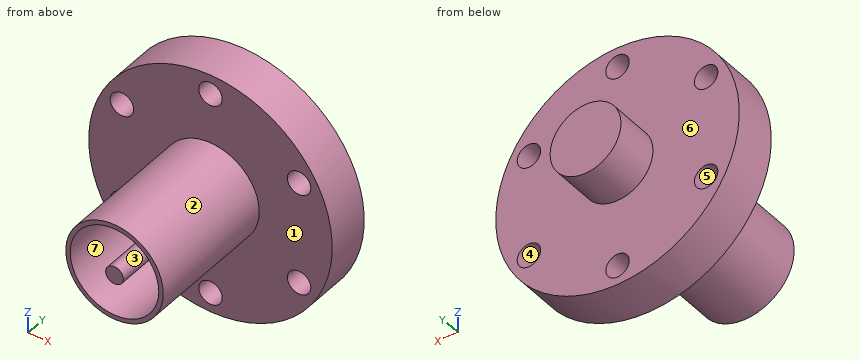
```python
from build123d import *

# Parameters (mm, degrees)
SKETCH1_R           = 34.925
EXTRUDE1_DEPTH      = 12.7
SKETCH3_R           = 3.3655
CUT_EXTRUDE2_DEPTH  = 12.7
CIRPATTERN1_COUNT   = 6
SKETCH6_R           = 10.16
EXTRUDE2_DEPTH      = 12.7
SKETCH7_R           = 13.97
SKETCH7_R_2         = 12.7
EXTRUDE_THIN2_DEPTH = 38.1
SKETCH8_R           = 2.54
EXTRUDE4_DEPTH      = 38.1


with BuildPart() as part:
    # Sketch1 → Extrude1 (new body)
    with BuildSketch(Plane(origin=(0, 0, 0), x_dir=(1, 0, 0), z_dir=(0, 1, 0))):
        with Locations(Location((0, 0, 0), (0, 0, 270))):
            Circle(SKETCH1_R)
    extrude(amount=EXTRUDE1_DEPTH)

    # Sketch3 → Cut-Extrude2 (cut)
    with BuildSketch(Plane(origin=(0, 0, 0), x_dir=(1, 0, 0), z_dir=(0, 1, 0))):
        with Locations(Location((0, 29.337, 0), (0, 0, 270))):
            Circle(SKETCH3_R)
    cut_extrude2 = extrude(amount=CUT_EXTRUDE2_DEPTH, mode=Mode.SUBTRACT)

    # CirPattern1: Cut-Extrude2 ×6 about axis
    cirpattern1_axis = Axis((0, 0, 0), (0, 1, 0))
    for i in range(1, CIRPATTERN1_COUNT):
        add(cut_extrude2.rotate(cirpattern1_axis, i * 360 / CIRPATTERN1_COUNT), mode=Mode.SUBTRACT)

    # Sketch6 → Extrude2 (add)
    with BuildSketch(Plane(origin=(0, 12.7, 0), x_dir=(-1, 0, 0), z_dir=(0, 1, 0))):
        with Locations(Location((0, 0, 0), (0, 0, 90))):
            Circle(SKETCH6_R)
    extrude(amount=EXTRUDE2_DEPTH)

    # Sketch7 → Extrude-Thin2 (add)
    with BuildSketch(Plane.XZ):
        with Locations((0, 0.982903874)):
            Circle(SKETCH7_R)
        with Locations((0, 0.982903874)):
            Circle(SKETCH7_R_2, mode=Mode.SUBTRACT)
    extrude(amount=EXTRUDE_THIN2_DEPTH)

    # Sketch8 → Extrude4 (add)
    with BuildSketch(Plane.XZ):
        with Locations(Location((0, 0, 0), (0, 0, 90))):
            Circle(SKETCH8_R)
    extrude(amount=EXTRUDE4_DEPTH)


solid = part.part
```
CAD build for the part. Positions are in the model's coordinates, mm. Face numbers are marked on the shaded views. A direction names the side the tool comes from. Give positions to 0.01 mm unless a question says otherwise; leave off trailing zeros. Order: outer loops, then holes, each group sorted by start corner. A loop starts at its lowest first (then second) coordinate and runs counter-clockwise, first axis right, second up.
(1) Mould opens along X. For the marked faces 1, 2, 3 and 4 say: released by +X, released by -X, zero draft, split by the parting line, or undercut.
(2) Tool access for the marked faces 5, 6 and 7: list every direction of +Z, -Z, +X, -X, +Y, -Y with a clear straight run to the whole face (end or side of a thin tool).
(3) Drill centre lines: L1, parallel to Z at x = 0.5, y = 12; L2, parallel to X at y = -25, z = -9; L3, parallel to Y at x = -6.5, z = -25. Where is each one in solid material? Low to high.
(4) Saw through at C-C, the plane z = -15. Give the cut face in (x, y), then the cut area to 3 significant figures.
(5) Saw through at B-B, the plane y = 11.5. State how many separate pieces and enclosed holes the cut face has, then the cut area to 3 significant figures.
(6) Saw through at D-D, the plane y = -17.5. Give the cut face in (x, z), then the cut area to 3 significant figures.
(7) Saw through at A-A, the plane x = 0. Give the cut face in (y, z) (1 decimal).
(8) Flat gauge pins, fed straight in: pin 1 (7.5 mm diameter, centred on x = 25.41, z = -14.67, fed in from +Y); pin 2 (6 mm diameter, centred on x = 19.5, y = 5.5, fed in from +Z); pin 3 (2 mm diameter, centred on x = -22.5, y = -0.5, fed in from -Z); pin 4 (4 mm diameter, centred on x = -25.41, z = -14.67, fed in from -Y). Where does each tip first touch, or does it go through?
Results found:
1. face 1: zero draft
1. face 2: split by the parting line
1. face 3: undercut
1. face 4: undercut
2. face 5: +Y, -Y
2. face 6: +Y
2. face 7: -Y
3. L1: z = -34.92 to -32.67, -26.01 to 26.01, 32.67 to 34.92
3. L2: x = -9.77 to -7.85, 7.85 to 9.77
3. L3: y = 0 to 12.7
4. outline: (-31.54, 0) - (-28.76, 0) - (-28.76, 12.7) - (-31.54, 12.7) - close; (-22.06, 0) - (22.06, 0) - (22.06, 12.7) - (-22.06, 12.7) - close; (28.76, 0) - (31.54, 0) - (31.54, 12.7) - (28.76, 12.7) - close
4. area: 631 mm2
5. separate pieces: 1
5. enclosed holes: 6
5. area: 3,620 mm2
6. outline: circle Ø27.94 at (0, 0.98); circle Ø5.08 at (0, 0); hole circle Ø25.4 at (0, 0.98)
6. area: 127 mm2
7. outline: (-38.1, -13) - (0, -13) - (0, -26) - (12.7, -26) - (12.7, -10.2) - (25.4, -10.2) - (25.4, 10.2) - (12.7, 10.2) - (12.7, 26) - (0, 26) - (0, 15) - (-38.1, 15) - (-38.1, 13.7) - (0, 13.7) - (0, 2.5) - (-38.1, 2.5) - (-38.1, -2.5) - (0, -2.5) - (0, -11.7) - (-38.1, -11.7) - close; (0, -34.9) - (12.7, -34.9) - (12.7, -32.7) - (0, -32.7) - close; (0, 32.7) - (12.7, 32.7) - (12.7, 34.9) - (0, 34.9) - close
8. pin 1: stops at y = 12.7
8. pin 2: stops at z = 30.78
8. pin 3: stops at z = -27.42
8. pin 4: passes through
